```python
from build123d import *

# Parameters (mm, degrees)
SKETCH_R         = 40.2
SKETCH_R_2       = 30
PAD_DEPTH        = 5
HOLE_D           = 3.6
HOLE_DEPTH       = 5
HOLE_CBORE_D     = 6.2
HOLE_CBORE_DEPTH = 3
CHAMFER_SIZE     = 0.4


with BuildPart() as part:
    # Sketch → Pad (new body)
    with BuildSketch(Plane.XY):
        Circle(SKETCH_R)
        Circle(SKETCH_R_2, mode=Mode.SUBTRACT)
    extrude(amount=PAD_DEPTH)

    # Hole
    with Locations(Plane.XY.offset(5)):
        with Locations((-36.6, 0), (18.3, 31.69653), (18.3, -31.69653)):
            CounterBoreHole(HOLE_D / 2, HOLE_CBORE_D / 2, HOLE_CBORE_DEPTH, depth=HOLE_DEPTH)

    # Chamfer
    chamfer_edges = [part.edges().sort_by_distance(p)[0] for p in [
        (-40.2, 0, 5),
        (-30, 0, 5),
        (-40.2, 0, 0),
        (-30, 0, 0),
    ]]
    chamfer(chamfer_edges, length=CHAMFER_SIZE)


solid = part.part
```
Can you work these out from the model? Positions are in its coordinate system, mm. A direction names the side the tool comes from. Give positions to 0.01 mm unless a question says otherwise; leave off trailing zeros. Order: outer loops, then holes, each group sorted by start corner. A loop starts at its lowest first (then second) coordinate and runs counter-clockwise, first axis right, second up. Notation, with made-up numbers: (27, -40) - (84, -40) arc R23 ccw to (84, -6) - close; hole circle Ø8 at (19, -38.75). An arc over 180 degrees is marked (long way). Use a Markdown table: item, result. Add a question column.
Q1. If we section it at D-D on x = 18.3: Count the separate pieces of the cut face and the enclosed holes in it, plus the area to 3 significant figures.
Q2. Please list where these lines run through material, in increasing order: line 1 along Y through (x, z) = (0, 1.35); line 2 along Y through (x, z) = (18.3, 1.35); line 3 along X through (y, z) = (1.5, 3.4).
Q3. If we mould it in two halves opening along Y, with no side actions, what happens to faces 3 (the cylindrical face through (15.84, 29.81, 3.52)), 4 (the flat face through (-9, -29.3, 0)), 5 (the cylindrical face through (38.344, 12.075, 2.471))? For each: released by +Y, released by -Y, zero draft, split by the parting line, or undercut.
Q4. If we section it at A-A on x = 0: Write out the boundary of the cut face in (y, z), plus the area to 3 significant figures.
Q5. If we section it at C-C on z = 3.65: Write out the boundary of the cut face in (x, y), plus the area to 3 significant figures.
Q6. On a 3-axis mill with a long thin cutter (end or side, diameter ignored), from which of +Z, -Z, +X, -X, +Y, -Y can I reach the whole of each face in a straight line? I mean faces 1 (the cylindrical face through (-39.7, 0.1, 3.5)), 2 (the flat face through (-30, -9, 5)). Say none if no direction works.
Q7. If we section it at B-B on y = 0: Write out the boundary of the cut face in (x, z), plus the area to 3 significant figures.
Q8. I'm going to push flat-ended pins straight in: pin 1 (3 mm diameter, centred on x = 18.3, y = -31.7, fed in from -Z); pin 2 (1 mm diameter, centred on x = -19.5, z = 1.5, fed in from +Y); pin 3 (2 mm diameter, centred on x = -30.5, z = 2.5, fed in from +Y); pin 4 (4 mm diameter, centred on x = -36.6, y = 0, fed in from +Z). Where does each tip first touch, or does it pass through?
Answers follow:
| question | item | result |
|---|---|---|
| 1 | separate pieces | 4 |
| 1 | enclosed holes | 0 |
| 1 | area | 67.8 mm^2 |
| 2 | line 1 | y = -40.2 to -30, 30 to 40.2 |
| 2 | line 2 | y = -35.79 to -33.5, -29.9 to -23.77, 23.77 to 29.9, 33.5 to 35.79 |
| 2 | line 3 | x = -40.17 to -39.31, -33.89 to -29.96, 29.96 to 40.17 |
| 3 | face 3 | undercut |
| 3 | face 4 | zero draft |
| 3 | face 5 | split by the parting line |
| 4 | outline | (-40.2, 0.4) - (-39.8, 0) - (-30.4, 0) - (-30, 0.4) - (-30, 4.6) - (-30.4, 5) - (-39.8, 5) - (-40.2, 4.6) - close; (30, 0.4) - (30.4, 0) - (39.8, 0) - (40.2, 0.4) - (40.2, 4.6) - (39.8, 5) - (30.4, 5) - (30, 4.6) - close |
| 4 | area | 101 mm^2 |
| 5 | outline | circle Ø80.4 at (0, 0); hole circle Ø6.2 at (-36.6, 0); hole circle Ø60 at (0, 0); hole circle Ø6.2 at (18.3, -31.7); hole circle Ø6.2 at (18.3, 31.7) |
| 5 | area | 2,160 mm^2 |
| 6 | face 1 | +Z |
| 6 | face 2 | +Z, +X, -X, +Y, -Y |
| 7 | outline | (-40.2, 0.4) - (-39.8, 0) - (-38.4, 0) - (-38.4, 2) - (-39.7, 2) - (-39.7, 5) - (-39.8, 5) - (-40.2, 4.6) - close; (-34.8, 0) - (-30.4, 0) - (-30, 0.4) - (-30, 4.6) - (-30.4, 5) - (-33.5, 5) - (-33.5, 2) - (-34.8, 2) - close; (30, 0.4) - (30.4, 0) - (39.8, 0) - (40.2, 0.4) - (40.2, 4.6) - (39.8, 5) - (30.4, 5) - (30, 4.6) - close |
| 7 | area | 75.6 mm^2 |
| 8 | pin 1 | passes through |
| 8 | pin 2 | stops at y = 35.43 |
| 8 | pin 3 | stops at y = 27.31 |
| 8 | pin 4 | stops at z = 2 |
